Could you check a few things on this model? Use its own coordinates, in mm. A direction names the side the tool comes from. Give positions to 0.01 mm unless a question says otherwise; leave off trailing zeros. Loops run counter-clockwise (first coordinate to the right, second up) from the corner with the lowest first, then second, coordinate; pieces in that order, holes last. Notation, with made-up numbers: (-35, 2) - (14, 2) arc R18 ccw to (14, 29) - close; hole circle Ø6 at (11.5, -29). An arc over 180 degrees is marked (long way). Use CSV: the item, a comma, the result in double quotes.
Solid Edge part; units mm, degrees
sketch "Sketch1" plane through (0, 0, 0) normal (0, 0, 1) x (1, 0, 0)
  circle A0 centre (0, 0) radius 2.75
extrude "Protrusion1" add sketch "Sketch1" along normal blind 3
sketch "Sketch2" plane through (0, 0, 3) normal (0, 0, 1) x (0, 1, 0)
  line L0 (0, 1.4434) -> (1.25, 0.7217)
  line L1 (1.25, 0.7217) -> (1.25, -0.7217)
  line L2 (1.25, -0.7217) -> (0, -1.4434)
  line L3 (0, -1.4434) -> (-1.25, -0.7217)
  line L4 (-1.25, -0.7217) -> (-1.25, 0.7217)
  line L5 (-1.25, 0.7217) -> (0, 1.4434)
extrude "Cutout1" cut sketch "Sketch2" against normal blind 1.3
fillet "Round1" radius 0.3 1 edges at (-2.75, 0, 3)
sketch "Sketch3" plane through (0, 0, 0) normal (1, 0, 0) x (0, 1, 0)
  line L0 (-1.1935, -16) -> (0, -16)
  line L1 (-1.5, -15.6935) -> (-1.1935, -16)
  line L2 (-1.5, -1.5) -> (-1.5, -15.6935)
  line L3 (-1.1935, -1.5) -> (-1.5, -1.5)
  line L4 (-1.1935, -1.49) -> (-1.1935, -1.5)
  line L5 (-1.5, -1.49) -> (-1.1935, -1.49)
  line L6 (-1.5, -0.1) -> (-1.5, -1.49)
  arc A0 (-1.5, -0.1) -> (-1.6, 0) centre (-1.6, -0.1) ccw
revolve "RevolvedProtrusion1" add sketch "Sketch3" angle 360 about axis through (0, 0, -60.325) along (0, 0, 1) material side at (0, -0.5968, -15.95)
cosmetic_thread "Thread1"
sketch "Sketch4" plane through (0, 0, 0) normal (0, -1, 0) x (1, 0, 0)
  line L0 (-1.435, 3) -> (0, 2.1715)
revolve "RevolvedCutout1" cut sketch "Sketch4" angle 360 about axis through (0, 0, 57.15) along (0, 0, -1) material side at (-0.6925, 0, 2.6291)
properties material "Stahl"
1) We'd pull the mould along X, two halves only. Please class faces 1 (the flat face through (0, -1.25, 2)), 2 (the cylindrical face through (-0.596, 2.685, 1.331)), 3 (the flat face through (2, 0, 0)): +X half, -X half, draft (parallel to the pull), parting line (faces both ways), or undercut.
Answer below:
face 1,"undercut"
face 2,"parting line"
face 3,"draft"
2) Which directions (+Z, -Z, +X, -X, +Y, -Y) give clear straight access to the entire face, cutting with the end or side of a thin tool? Please do faces 4 (the flat face through (0, 0, -16)), 5 (the flat face through (1.088, -0.616, 2.359)), 6 (the cylindrical face through (-0.07, 1.5, -8.7)).
Answer below:
face 4,"-Z, +X, -X, +Y, -Y"
face 5,"+Z"
face 6,"-Z"
3) Suppose I cut it at C-C (z = -10.25). Please give me the cut outline in (x, y), plus the area to 3 significant figures.
Answer below:
outline,"circle Ø3 at (0, 0)"
area,"7.07 mm2"
4) Suppose I cut it at B-B (z = 0.5). Please give me the cut outline in (x, y).
Answer below:
outline,"circle Ø5.5 at (0, 0)"
5) I need wall thicknesses on line 1 along Z through (x, y) = (-0.1, 0.05); line 2 along Z through (x, y) = (1.6, 0.35); line 3 along X through (y, z) = (-1.1, -8.75). Which ranges of each line are inside material? Lowest first, please.
Answer below:
line 1,"z = -16 to 1.7"
line 2,"z = 0 to 3"
line 3,"x = -1.02 to 1.02"
